Verification items for the finished model (mm, model axes). Coordinates: 2 decimals unless noted, no trailing zeros. Write each loop counter-clockwise with the first axis right and the second up, starting at its lowest first coordinate (ties: lowest second). Pieces come first, ordered by that corner, then holes. Notation, with made-up numbers: M 66,45.25 L 115,45.25 A19 ccw 115,60.25 Z; hole C -5,49.5 d1. An arc over 180 degrees is marked long. Answer in a Markdown table with one row per item.
from build123d import *

# Parameters (mm, degrees)
SKETCH1_R                   = 12.7
BOSS_EXTRUDE1_DEPTH         = 20.955
SKETCH2_R                   = 1.24968
CUT_EXTRUDE1_DEPTH          = 25.4
CIRPATTERN1_COUNT           = 3
CIRPATTERN2_COUNT           = 2
CIRPATTERN2_ANGLE           = 30
CIRPATTERN2_COPY_1_SKETCH_R = 1.24968
CIRPATTERN2_COPY_1_DEPTH    = 25.4
CIRPATTERN2_COPY_2_SKETCH_R = 1.24968
CIRPATTERN2_COPY_2_DEPTH    = 25.4


with BuildPart() as part:
    # Sketch1 → Boss-Extrude1 (new body)
    with BuildSketch(Plane.XY):
        Circle(SKETCH1_R)
    extrude(amount=BOSS_EXTRUDE1_DEPTH)

    # Sketch2 → Cut-Extrude1 (cut)
    with BuildSketch(Plane(origin=(0, 0, 0), x_dir=(-1, 0, 0), z_dir=(0, 0, -1))):
        with Locations((0, 10.16)):
            Circle(SKETCH2_R)
    cut_extrude1 = extrude(amount=-CUT_EXTRUDE1_DEPTH, mode=Mode.SUBTRACT)

    # CirPattern1: Cut-Extrude1 ×3 about axis
    cirpattern1_axis = Axis((0, 0, 0), (0, 0, 1))
    for i in range(1, CIRPATTERN1_COUNT):
        add(cut_extrude1.rotate(cirpattern1_axis, i * 360 / CIRPATTERN1_COUNT), mode=Mode.SUBTRACT)

    # CirPattern2: Cut-Extrude1 ×2 about axis
    cirpattern2_axis = Axis((0, 0, 0), (0, 0, 1))
    for i in range(1, CIRPATTERN2_COUNT):
        add(cut_extrude1.rotate(cirpattern2_axis, i * CIRPATTERN2_ANGLE / (CIRPATTERN2_COUNT - 1)), mode=Mode.SUBTRACT)

    # CirPattern2 copy 1 sketch → CirPattern2 copy 1 (cut)
    with BuildSketch(Plane(origin=(0, 0, 0), x_dir=(0.8660254037844392, -0.4999999999999991, 0), z_dir=(0, 0, -1))):
        with Locations((0, 10.16)):
            Circle(CIRPATTERN2_COPY_1_SKETCH_R)
    extrude(amount=-CIRPATTERN2_COPY_1_DEPTH, mode=Mode.SUBTRACT)

    # CirPattern2 copy 2 sketch → CirPattern2 copy 2 (cut)
    with BuildSketch(Plane.YX):
        with Locations((0, 10.16)):
            Circle(CIRPATTERN2_COPY_2_SKETCH_R)
    extrude(amount=-CIRPATTERN2_COPY_2_DEPTH, mode=Mode.SUBTRACT)


solid = part.part
1) Depth check by flat-ended pin: pin 1 (1.5 mm diameter, centred on y = 3, z = 9, fed in from -X); pin 2 (3 mm diameter, centred on y = 10, z = 17.5, fed in from -X); pin 3 (4 mm diameter, centred on x = 3.5, z = 13.5, fed in from +Y); pin 4 (1.5 mm diameter, centred on x = 8.8, y = -5.08, fed in from +Z). Enter the tip coordinate at first touch or a pass-through.
Response values:
| item | result |
|---|---|
| pin 1 | stops at x = -12.5 |
| pin 2 | stops at x = -9.44 |
| pin 3 | stops at y = 12.61 |
| pin 4 | passes through |
2) Sectioned sample at D-D (x = -5.08). Record the cut outline in (y, z) (1 decimal).
Response values:
| item | result |
|---|---|
| outline | M -11.6,0 L -10,0 L -10,21 L -11.6,21 Z; M -7.5,0 L 7.5,0 L 7.5,21 L -7.5,21 Z; M 10,0 L 11.6,0 L 11.6,21 L 10,21 Z |
3) Sectioned sample at A-A (y = 0). Record the cut outline in (x, z) (3 decimals), then the cut area to 3 significant figures.
Response values:
| item | result |
|---|---|
| outline | M -12.7,0 L 8.91,0 L 8.91,20.955 L -12.7,20.955 Z; M 11.41,0 L 12.7,0 L 12.7,20.955 L 11.41,20.955 Z |
| area | 480 mm² |
4) Sectioned sample at C-C (z = 12.25). Record the cut outline in (x, y), then the cut area to 3 significant figures.
Response values:
| item | result |
|---|---|
| outline | C 0,0 d25.4; hole C -8.8,-5.08 d2.5; hole C -5.08,-8.8 d2.5; hole C -5.08,8.8 d2.5; hole C 0,10.16 d2.5; hole C 8.8,-5.08 d2.5; hole C 10.16,0 d2.5 |
| area | 477 mm² |
5) Thickness scan on L1, parallel to Y at x = 0, z = 6.75; L2, parallel to X at y = -5.25, z = 13.5; L3, parallel to X at y = -8.25, z = 6.75. Record the ranges inside material, lowest first. Write a range as [from, to].
Response values:
| item | result |
|---|---|
| L1 | y = [-12.7, 8.91], [11.41, 12.7] |
| L2 | x = [-11.56, -10.04], [-7.56, 7.56], [10.04, 11.56] |
| L3 | x = [-9.66, -6.2], [-3.96, 9.66] |
6) Release check for a two-part mould opening along X. For faces 1 (the face through (0, 0, 20.955)), 2 (the face through (-2.75, -12.4, 10.33)), 3 (the face through (-9.375, -6.189, 10.331)) record: +X half, -X half, draft (parallel to the pull), parting line (faces both ways), or undercut.
Response values:
| item | result |
|---|---|
| face 1 | draft |
| face 2 | parting line |
| face 3 | undercut |
